The model under review builds one solid part; all positions refer to its coordinate system, in mm. Face numbers are marked on the shaded views. Give positions to 0.01 mm unless a question says otherwise; leave off trailing zeros. Loops run counter-clockwise (first coordinate to the right, second up) from the corner with the lowest first, then second, coordinate; pieces in that order, holes last. Notation, with made-up numbers: M -39.5,-27.75 L -21.5,-27.75 A24 cw -21.5,-2.75 Z; hole C 47.5,-22 d9. An arc over 180 degrees is marked long. Return JSON: item names as keys, results as strings.
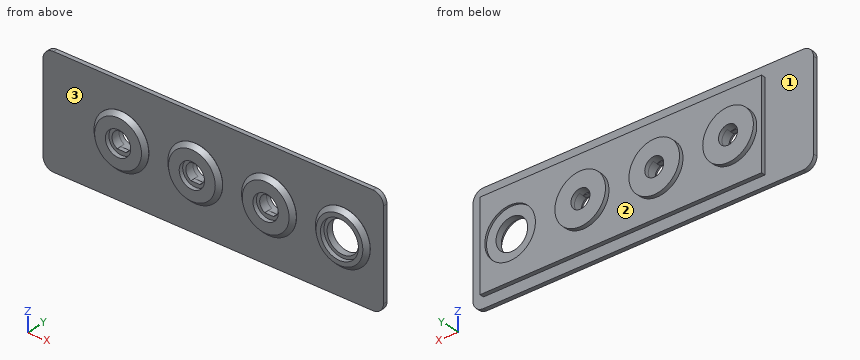
```python
from build123d import *

# Parameters (mm, degrees)
SKETCH_W               = 133.5
SKETCH_H               = 42
PAD_DEPTH              = 2
SKETCH001_W            = 161.5
SKETCH001_H            = 52
PAD001_DEPTH           = 2
SKETCH002_R            = 7.5
POCKET_DEPTH           = 4.001
SKETCH003_R            = 12
POCKET001_DEPTH        = 1
SKETCH004_R            = 12
PAD002_DEPTH           = 2
SKETCH005_R            = 4.5
POCKET002_DEPTH        = 4
LINEARPATTERN_COUNT    = 3
LINEARPATTERN_PITCH    = 35
SKETCH006_R            = 13
SKETCH006_R_2          = 6
PAD003_DEPTH           = 2
LINEARPATTERN001_COUNT = 3
LINEARPATTERN001_PITCH = 35
CHAMFER_SIZE           = 1.9
FILLET_R               = 5
SKETCH007_R            = 13
SKETCH007_R_2          = 9
PAD004_DEPTH           = 2
CHAMFER001_SIZE        = 1.9


with BuildPart() as part:
    # Sketch → Pad (new body)
    with BuildSketch(Plane.XZ):
        with Locations((66.75, 21)):
            Rectangle(SKETCH_W, SKETCH_H)
    extrude(amount=PAD_DEPTH)

    # Sketch001 (on Face6 of Pad) → Pad001 (join)
    with BuildSketch(Plane.XZ.offset(2)):
        with Locations((57.75, 21)):
            Rectangle(SKETCH001_W, SKETCH001_H)
    extrude(amount=PAD001_DEPTH)

    # Sketch002 (on Face11 of Pad001) → Pocket (cut, through all)
    with BuildSketch(Plane.XZ.offset(4)):
        with Locations((119.25, 21)):
            Circle(SKETCH002_R)
        with BuildLine():
            ThreePointArc((12.188447, 25), (9.75, 21), (12.188447, 17))
            Line((12.188447, 17), (16.311553, 17))
            ThreePointArc((16.311553, 17), (18.75, 21), (16.311553, 25))
            Line((12.188447, 25), (16.311553, 25))
        make_face()
        with BuildLine():
            ThreePointArc((47.188447, 25), (44.75, 21), (47.188447, 17))
            Line((47.188447, 17), (51.311553, 17))
            ThreePointArc((51.311553, 17), (53.75, 21), (51.311553, 25))
            Line((51.311553, 25), (47.188447, 25))
        make_face()
        with BuildLine():
            Line((82.188447, 17), (86.311553, 17))
            ThreePointArc((86.311553, 17), (88.75, 21), (86.311553, 25))
            Line((86.311553, 25), (82.188447, 25))
            ThreePointArc((82.188447, 25), (79.75, 21), (82.188447, 17))
        make_face()
    extrude(amount=-POCKET_DEPTH, mode=Mode.SUBTRACT)

    # Sketch003 (on Face1 of Pocket) → Pocket001 (cut)
    with BuildSketch(Plane(origin=(0, 0, 0), x_dir=(1, 0, 0), z_dir=(0, 1, 0))):
        with Locations((119.25, -21)):
            Circle(SKETCH003_R)
    extrude(amount=-POCKET001_DEPTH, mode=Mode.SUBTRACT)

    # Sketch004 (on Face1 of Pocket001) → Pad002 (join)
    with BuildSketch(Plane(origin=(0, 0, 0), x_dir=(1, 0, 0), z_dir=(0, 1, 0))):
        with Locations((84.355629, -21.002337)):
            Circle(SKETCH004_R)
        with Locations((49.25, -21)):
            Circle(SKETCH004_R)
        with Locations((14.25, -21.000002)):
            Circle(SKETCH004_R)
    extrude(amount=PAD002_DEPTH)

    # Sketch005 (on Face17 of Pad002) → Pocket002 (cut)
    with BuildSketch(Plane(origin=(0, 2, 0), x_dir=(1, 0, 0), z_dir=(0, 1, 0))):
        with Locations((14.25, -21)):
            Circle(SKETCH005_R)
        with Locations((49.25, -21)):
            Circle(SKETCH005_R)
        with Locations((84.25, -21)):
            Circle(SKETCH005_R)
    pocket002 = extrude(amount=-POCKET002_DEPTH, mode=Mode.SUBTRACT)

    # LinearPattern: Pocket002 ×3
    with Locations(*[(-i * LINEARPATTERN_PITCH, 0, 0) for i in range(1, LINEARPATTERN_COUNT)]):
        add(pocket002, mode=Mode.SUBTRACT)

    # Sketch006 (on Face19 of LinearPattern) → Pad003 (join)
    with BuildSketch(Plane.XZ.offset(4)):
        with Locations((84.25, 21)):
            Circle(SKETCH006_R)
        with Locations((84.25, 21)):
            Circle(SKETCH006_R_2, mode=Mode.SUBTRACT)
    pad003 = extrude(amount=PAD003_DEPTH)

    # LinearPattern001: Pad003 ×3
    with Locations(*[(-i * LINEARPATTERN001_PITCH, 0, 0) for i in range(1, LINEARPATTERN001_COUNT)]):
        add(pad003)

    # Chamfer
    chamfer_edges = [part.edges().sort_by_distance(p)[0] for p in [
        (1.25, -6, 21),
        (36.25, -6, 21),
        (71.25, -6, 21),
    ]]
    chamfer(chamfer_edges, length=CHAMFER_SIZE)

    # Fillet
    fillet_edges = [part.edges().sort_by_distance(p)[0] for p in [
        (-23, -3, -5),
        (-23, -3, 47),
        (138.5, -3, -5),
        (138.5, -3, 47),
    ]]
    fillet(fillet_edges, radius=FILLET_R)

    # Sketch007 (on Face1 of Fillet) → Pad004 (join)
    with BuildSketch(Plane.XZ.offset(4)):
        with Locations((119.25, 21)):
            Circle(SKETCH007_R)
        with Locations((119.25, 21)):
            Circle(SKETCH007_R_2, mode=Mode.SUBTRACT)
    extrude(amount=PAD004_DEPTH)

    # Chamfer001
    chamfer001_edges = [part.edges().sort_by_distance(p)[0] for p in [
        (106.25, -6, 21),
    ]]
    chamfer(chamfer001_edges, length=CHAMFER001_SIZE)


solid = part.part
```
1) Insertion check: pin 1 (1 mm diameter, centred on x = 97, z = 9.5, fed in from +Y); pin 2 (12 mm diameter, centred on x = 63, z = 33.5, fed in from -Y); pin 3 (7 mm diameter, centred on x = 14.25, z = 21, fed in from -Y); pin 4 (1 mm diameter, centred on x = 97, y = -1, fed in from -Z). Each pin has a flat end and moves straight along its axis. Give the tip position at first contact, or say it passes through.
From the geometry:
{"pin 1": "y = 0", "pin 2": "y = -4.52", "pin 3": "through", "pin 4": "z = 0"}
2) Wall thickness on L1, parallel to X at y = -0.35, z = 21; L2, parallel to Z at x = 84.25, y = -5.1; L3, parallel to X at y = -1.25, z = 19.5: over which ranges is each line inside the solid? List them lowest first. Write a range as from..to.
From the geometry:
{"L1": "0..9.75, 18.75..44.75, 53.75..79.75, 88.75..107.25, 131.25..133.5", "L2": "9..15, 27..33", "L3": "0..10.01, 18.49..45.01, 53.49..80.01, 88.49..111.9, 126.6..133.5"}
3) The part is to be moulded in two halves that separate along X. For the marked faces 1, 2 and 3, say which applies: released by +X, released by -X, zero draft, split by the parting line, or undercut.
From the geometry:
{"face 1": "zero draft", "face 2": "undercut", "face 3": "undercut"}
4) Consider section B-B on z = 39. Write out the cut boundary in (x, y), then the cut area to 3 significant figures.
From the geometry:
{"outline": "M -23,-4 L 138.5,-4 L 138.5,-2 L 133.5,-2 L 133.5,0 L 0,0 L 0,-2 L -23,-2 Z", "area": "590 mm²"}
5) Consider section C-C on x = 30. Write out the cut boundary in (y, z).
From the geometry:
{"outline": "M -4,-5 L -2,-5 L -2,0 L 0,0 L 0,42 L -2,42 L -2,47 L -4,47 Z"}
6) Consider section D-D on z = 19. Count the separate pieces of the cut face and the enclosed holes in it, then the cut area to 3 significant figures.
From the geometry:
{"separate pieces": "5", "enclosed holes": "0", "area": "608 mm²"}
